Work out the finished part from the listing and answer in its coordinate system (mm). A direction names the side the tool comes from. Coordinates: 2 decimals unless noted, no trailing zeros. Order: outer loops, then holes, each group sorted by start corner. A loop starts at its lowest first (then second) coordinate and runs counter-clockwise, first axis right, second up. Notation, with made-up numbers: M 69.25,42 L 117.25,42 A25 ccw 117.25,72 Z; hole C 14,-28 d2. An arc over 180 degrees is marked long. Use a Markdown table: item, result.
from build123d import *

# Parameters (mm, degrees)
SKETCH1_R           = 60.325
BOSS_EXTRUDE1_DEPTH = 12.7
SKETCH2_R           = 3.175
CUT_EXTRUDE1_DEPTH  = 19.05
CRVPATTERN1_COUNT   = 5


with BuildPart() as part:
    # Sketch1 → Boss-Extrude1 (new body)
    with BuildSketch(Plane(origin=(0, 0, 0), x_dir=(1, 0, 0), z_dir=(0, 1, 0))):
        with Locations(Location((0, 0, 0), (0, 0, 270))):
            Circle(SKETCH1_R)
    extrude(amount=BOSS_EXTRUDE1_DEPTH)

    # Sketch2 → Cut-Extrude1 (cut)
    with BuildSketch(Plane.XY.offset(76.2)):
        with Locations((0, 6.35)):
            Circle(SKETCH2_R)
    cut_extrude1 = extrude(amount=-CUT_EXTRUDE1_DEPTH, mode=Mode.SUBTRACT)

    # CrvPattern1: Cut-Extrude1 ×5 about axis
    crvpattern1_axis = Axis((0, 12.7, 0), (0, -1, 0))
    for i in range(1, CRVPATTERN1_COUNT):
        add(cut_extrude1.rotate(crvpattern1_axis, i * 360 / CRVPATTERN1_COUNT), mode=Mode.SUBTRACT)


solid = part.part
1. Section C-C on z = -12 is taken. Determine the outline of the cut face in (x, y), then the cut area to 3 significant figures.
Answers below:
| item | result |
|---|---|
| outline | M -59.12,0 L 59.12,0 L 59.12,12.7 L -59.12,12.7 Z |
| area | 1,500 mm² |
2. Flat-ended cylindrical pins translate along their axes: P1, Ø4, axis at y = 4, z = -39, coming from the -X side; P2, Ø1.5, axis at x = -13.5, y = 2.5, coming from the -Z side; P3, Ø6, axis at x = 19.5, y = 7, coming from the +Z side. Find the tip coordinate at first contact, or state that the pin passes through.
Answers below:
| item | result |
|---|---|
| P1 | x = -47.65 |
| P2 | z = -58.96 |
| P3 | z = 58.02 |
3. For a pull along X with two mould halves and no side action, classify faces 4 (the face through (33.63, 6.39, -46.21)), 5 (the face through (1, 12.7, -1)), 6 (the face through (18.12, 6.26, 57.54)) as +X half, -X half, draft (parallel to the pull), parting line (faces both ways), or undercut.
Answers below:
| item | result |
|---|---|
| face 4 | undercut |
| face 5 | draft |
| face 6 | parting line |
4. For faces 1 (the face through (1, 0, -1)), 2 (the face through (0, 6, 57.15)), 3 (the face through (-33.56, 6.39, -46.26)), determine the directions among +Z, -Z, +X, -X, +Y, -Y from which every point of the face is accessible in a straight line to the end or side of a thin tool.
Answers below:
| item | result |
|---|---|
| face 1 | +Z, -Z, +X, -X, -Y |
| face 2 | +Z |
| face 3 | none |
5. Find the intervals of material crossed by probe 1 along Y at (x, z) = (0, 58.75) (3 decimals); probe 2 along Z at (x, y) = (24, 2.75); probe 3 along X at (y, z) = (9.75, -34.5), in increasing order.
Answers below:
| item | result |
|---|---|
| probe 1 | 0 to 3.175, 9.525 to 12.7 |
| probe 2 | -55.35 to 55.35 |
| probe 3 | -49.49 to 49.49 |
6. Section B-B on z = -29.5 is taken. Determine the outline of the cut face in (x, y).
Answers below:
| item | result |
|---|---|
| outline | M -52.62,0 L 52.62,0 L 52.62,12.7 L -52.62,12.7 Z |
